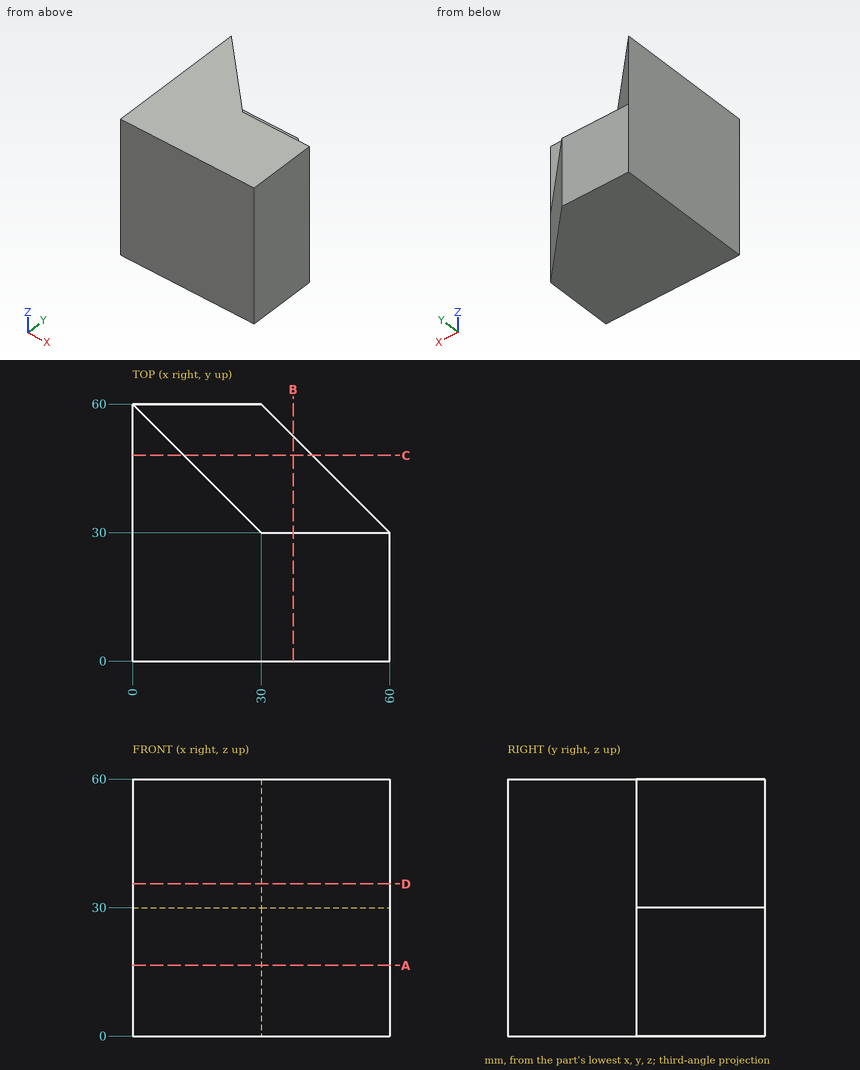
Geometry check sheet. Reference: drawing and pictorial views, mm from the part's lowest x, y, z. Round coordinates to 2 decimals unless told otherwise and drop trailing zeros. Loops run counter-clockwise (first coordinate to the right, second up) from the corner with the lowest first, then second, coordinate; pieces in that order, holes last. Notation, with made-up numbers: (-14, 87) -> (32, 87) arc R27 ccw to (32, 108) -> close; hole circle Ø2 at (-16, -11). An arc over 180 degrees is marked (long way). Answer as a JSON object with one key per item and string values. Group by question number.
Item 1: Thickness scan on line 1 along Z through (x, y) = (45.5, 43); line 2 along X through (y, z) = (31, 15). Record the ranges inside material, lowest first.
Item 2: Cross-section at C-C, the plane y = 48. Record the cut outline in (x, z).
Item 3: Cross-section at D-D, the plane z = 35.5. Record the cut outline in (x, y).
Item 4: Cross-section at B-B, the plane x = 37.5. Record the cut outline in (y, z).
Item 5: Depth check by flat-ended pin: pin 1 Ø15 at (x, y) = (32.5, 43) entering from +Z; pin 2 Ø12 at (y, z) = (52.5, 6.5) entering from +X; pin 3 Ø9 at (x, z) = (48.5, 50) entering from +Y. Enter the tip coordinate at first touch or a pass-through.
Item 6: Cross-section at A-A, the plane z = 16.5. Record the cut outline in (x, y).
Determined:
{
 "1": {"line 1": "z = 0 to 30", "line 2": "x = 0 to 59"},
 "2": {"outline": "(0, 0) -> (42, 0) -> (42, 30) -> (12, 30) -> (12, 60) -> (0, 60) -> close"},
 "3": {"outline": "(0, 0) -> (60, 0) -> (60, 30) -> (30, 30) -> (0, 60) -> close"},
 "4": {"outline": "(0, 0) -> (52.5, 0) -> (52.5, 30) -> (30, 30) -> (30, 60) -> (0, 60) -> close"},
 "5": {"pin 1": "stops at z = 30", "pin 2": "stops at x = 43.5", "pin 3": "stops at y = 30"},
 "6": {"outline": "(0, 0) -> (60, 0) -> (60, 30) -> (30, 60) -> (0, 60) -> close"}
}
